Part print with two shaded views. Sizes in mm from the minimum x, y, z corner. A direction names the side the tool comes from. Round coordinates to 2 decimals unless told otherwise and drop trailing zeros. Write each loop counter-clockwise with the first axis right and the second up, starting at its lowest first coordinate (ties: lowest second). Pieces come first, ordered by that corner, then holes.
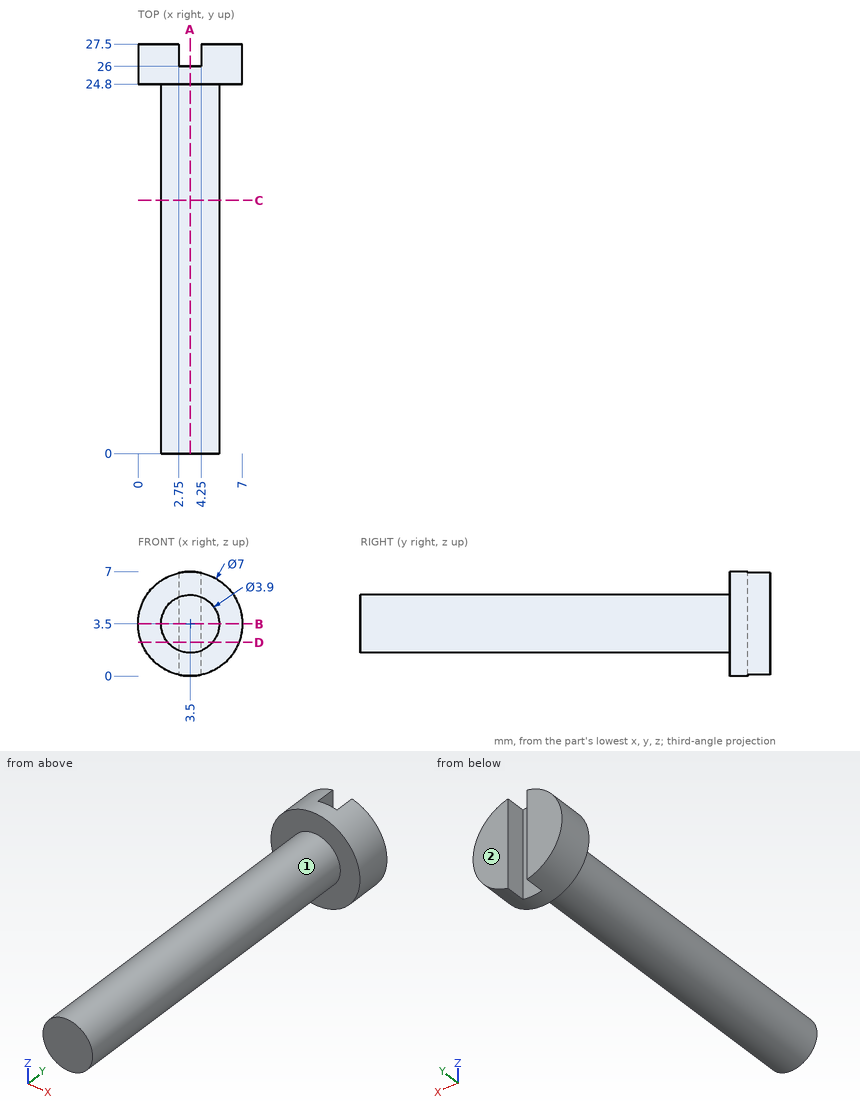
Q1. Cut at C-C on y = 17. Write the cut outline in (x, z).
Values follow:
outline: circle Ø3.9 at (3.5, 3.5)
Q2. Cut at D-D on z = 2.25. Write the cut outline in (x, y).
Values follow:
outline: (0.23, 24.8) - (2, 24.8) - (2, 0) - (5, 0) - (5, 24.8) - (6.77, 24.8) - (6.77, 27.5) - (4.25, 27.5) - (4.25, 26) - (2.75, 26) - (2.75, 27.5) - (0.23, 27.5) - close
Q3. Which spindle directions (+Z, -Z, +X, -X, +Y, -Y) get a long thin tool onto all of the face, cutting with end or side? Do the marked faces 1 and 2. Say none if no direction does.
Values follow:
face 1: -Y
face 2: +Z, -Z, +X, -X, +Y
Q4. Cut at A-A on x = 3.5. Write the cut outline in (y, z).
Values follow:
outline: (0, 1.55) - (24.8, 1.55) - (24.8, 0) - (26, 0) - (26, 7) - (24.8, 7) - (24.8, 5.45) - (0, 5.45) - close
Q5. Drop flat-ended pins along their axis: pin 1 (1.5 mm diameter, centred on y = 4, z = 4.5, fed in from +X); pin 2 (3 mm diameter, centred on x = 3, y = 6, fed in from -Z); pin 3 (0.8 mm diameter, centred on x = 3.5, z = 3, fed in from +Y). Give the stop position or say it passes through.
Values follow:
pin 1: stops at x = 5.43
pin 2: stops at z = 1.55
pin 3: stops at y = 26
Q6. Cut at B-B on z = 3.5. Write the cut outline in (x, y).
Values follow:
outline: (0, 24.8) - (1.55, 24.8) - (1.55, 0) - (5.45, 0) - (5.45, 24.8) - (7, 24.8) - (7, 27.5) - (4.25, 27.5) - (4.25, 26) - (2.75, 26) - (2.75, 27.5) - (0, 27.5) - close
Q7. Wall check: L1, parallel to Y at x = 0.75, z = 4.25; L2, parallel to Z at x = 4.25, y = 14; L3, parallel to X at y = 5, z = 2. Give the ranges that are in metal, low to high.
Values follow:
L1: y = 24.8 to 27.5
L2: z = 1.7 to 5.3
L3: x = 2.25 to 4.75
